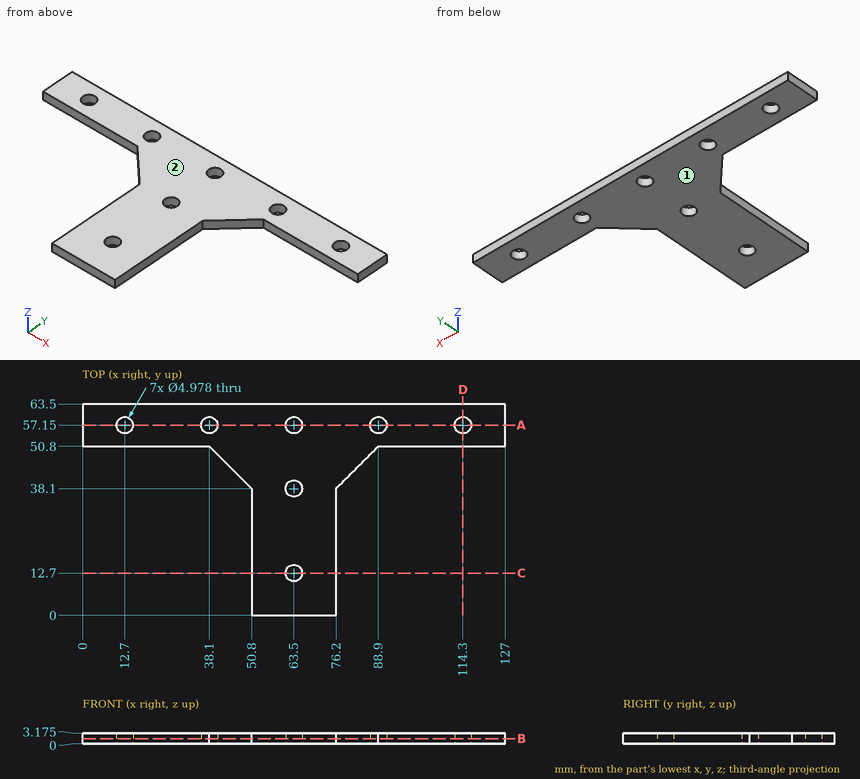
Can you work these out from the drawing? Everything is in mm from the part's minimum corner. Round coordinates to 2 decimals unless told otherwise and drop trailing zeros. Write each loop counter-clockwise with the first axis right and the second up, starting at its lowest first coordinate (ties: lowest second). Pieces come first, ordered by that corner, then holes. Notation, with made-up numbers: (-35.75, 81.5) - (-20.75, 81.5) arc R20 ccw to (-20.75, 97.5) - close; hole circle Ø9 at (48, -27.5). An arc over 180 degrees is marked (long way). Use a Markdown table: item, result.
Q1. Thinking about a two-plate mould opening in Z: for the marked faces 1 and 2, which applies, released by +Z, released by -Z, zero draft, split by the parting line, or undercut?
Output values:
| item | result |
|---|---|
| face 1 | released by -Z |
| face 2 | released by +Z |
Q2. Please list where these lines run through material, in increasing order: L1, parallel to Y at x = 63.5, z = 0.9; L2, parallel to X at y = 13, z = 2.2; L3, parallel to Y at x = 88.9, z = 2.1.
Output values:
| item | result |
|---|---|
| L1 | 0 to 10.21, 15.19 to 35.61, 40.59 to 54.66, 59.64 to 63.5 |
| L2 | 50.8 to 61.03, 65.97 to 76.2 |
| L3 | 50.8 to 54.66, 59.64 to 63.5 |
Q3. For pin 1 (1 mm diameter, centred on x = 28, z = 1, fed in from -Y); pin 2 (1.6 mm diameter, centred on y = 19.5, z = 1.5, fed in from -X), each with a flat end and sliding along its axis, tell me the tip position at first contact or that it passes through.
Output values:
| item | result |
|---|---|
| pin 1 | y = 50.8 |
| pin 2 | x = 50.8 |
Q4. I want a section at A-A (y = 57.15). List the corners of the cut face in (x, z) for me (1 decimal).
Output values:
| item | result |
|---|---|
| outline | (0, 0) - (10.2, 0) - (10.2, 3.2) - (0, 3.2) - close; (15.2, 0) - (35.6, 0) - (35.6, 3.2) - (15.2, 3.2) - close; (40.6, 0) - (61, 0) - (61, 3.2) - (40.6, 3.2) - close; (66, 0) - (86.4, 0) - (86.4, 3.2) - (66, 3.2) - close; (91.4, 0) - (111.8, 0) - (111.8, 3.2) - (91.4, 3.2) - close; (116.8, 0) - (127, 0) - (127, 3.2) - (116.8, 3.2) - close |
Q5. I want a section at D-D (x = 114.3). List the corners of the cut face in (y, z) for me (1 decimal), plus the area to 3 significant figures.
Output values:
| item | result |
|---|---|
| outline | (50.8, 0) - (54.7, 0) - (54.7, 3.2) - (50.8, 3.2) - close; (59.6, 0) - (63.5, 0) - (63.5, 3.2) - (59.6, 3.2) - close |
| area | 24.5 mm2 |
Q6. I want a section at B-B (z = 1.6). List the corners of the cut face in (x, y) for me.
Output values:
| item | result |
|---|---|
| outline | (0, 50.8) - (38.1, 50.8) - (50.8, 38.1) - (50.8, 0) - (76.2, 0) - (76.2, 38.1) - (88.9, 50.8) - (127, 50.8) - (127, 63.5) - (0, 63.5) - close; hole circle Ø4.98 at (12.7, 57.15); hole circle Ø4.98 at (38.1, 57.15); hole circle Ø4.98 at (63.5, 12.7); hole circle Ø4.98 at (63.5, 38.1); hole circle Ø4.98 at (63.5, 57.15); hole circle Ø4.98 at (88.9, 57.15); hole circle Ø4.98 at (114.3, 57.15) |
Q7. I want a section at C-C (y = 12.7). List the corners of the cut face in (x, z) for me (1 decimal).
Output values:
| item | result |
|---|---|
| outline | (50.8, 0) - (61, 0) - (61, 3.2) - (50.8, 3.2) - close; (66, 0) - (76.2, 0) - (76.2, 3.2) - (66, 3.2) - close |
